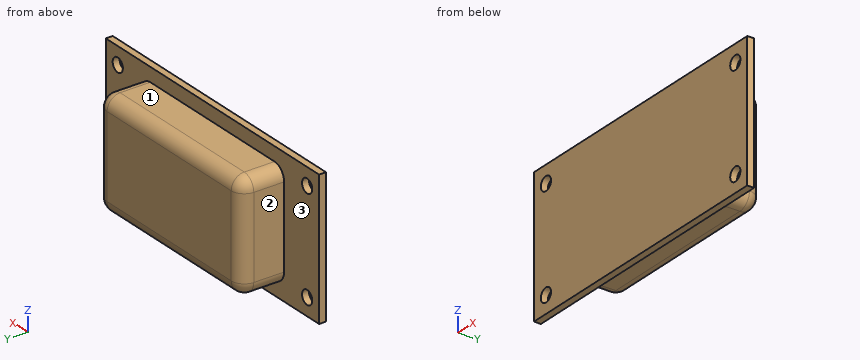
```python
from build123d import *

# Parameters (mm, degrees)
SKETCH_1_W      = 67
SKETCH_1_H      = 31.5
SKETCH_1_R      = 1.6
EXTRUDE_1_DEPTH = 1.6
SKETCH_2_W      = 45
SKETCH_2_H      = 25
EXTRUDE_2_DEPTH = 10
FILLET_1_R      = 3


with BuildPart() as part:
    # 草圖1 → 填料-伸長1 (new body)
    with BuildSketch(Plane(origin=(0, 0, 0), x_dir=(1, 0, 0), z_dir=(0, 1, 0))):
        Rectangle(SKETCH_1_W, SKETCH_1_H)
        with Locations(Location((-29.75, 11.75, 0), (0, 0, 270))):
            Circle(SKETCH_1_R, mode=Mode.SUBTRACT)
        with Locations(Location((-29.75, -11.75, 0), (0, 0, 270))):
            Circle(SKETCH_1_R, mode=Mode.SUBTRACT)
        with Locations(Location((29.75, -11.75, 0), (0, 0, 270))):
            Circle(SKETCH_1_R, mode=Mode.SUBTRACT)
        with Locations(Location((29.75, 11.75, 0), (0, 0, 270))):
            Circle(SKETCH_1_R, mode=Mode.SUBTRACT)
    extrude(amount=EXTRUDE_1_DEPTH)

    # 草圖2 → 填料-伸長2 (add)
    with BuildSketch(Plane(origin=(0, 1.6, 0), x_dir=(1, 0, 0), z_dir=(0, 1, 0))):
        Rectangle(SKETCH_2_W, SKETCH_2_H)
    extrude(amount=EXTRUDE_2_DEPTH)

    # 圓角1
    fillet_1_edges = [part.edges().sort_by_distance(p)[0] for p in [
        (22.5, 6.6, 12.5),
        (22.5, 6.6, -12.5),
        (-22.5, 6.6, -12.5),
        (-22.5, 6.6, 12.5),
        (22.5, 11.6, 0),
        (0, 11.6, -12.5),
        (-22.5, 11.6, 0),
        (0, 11.6, 12.5),
    ]]
    fillet(fillet_1_edges, radius=FILLET_1_R)


solid = part.part
```
Model file for the job. Use its own axes, mm. Face numbers are marked on the shaded views. A direction names the side the tool comes from. Coordinates: 2 decimals unless noted, no trailing zeros. Write each loop counter-clockwise with the first axis right and the second up, starting at its lowest first coordinate (ties: lowest second). Pieces come first, ordered by that corner, then holes. Notation, with made-up numbers: (2.5, -2) - (15.5, -2) arc R23 cw to (15.5, 11) - close; hole circle Ø9 at (-26.5, 16). An arc over 180 degrees is marked (long way). One line per item, written item: value. Start each with the question number.
1. Flat gauge pins, fed straight in: pin 1 (1 mm diameter, centred on y = 5, z = 4, fed in from +X); pin 2 (6 mm diameter, centred on x = 7.5, y = 7, fed in from -Z); pin 3 (5.5 mm diameter, centred on y = 5.5, z = -0.5, fed in from -X). Where does each tip first touch, or does it go through?
2. Slice it at A-A (x = 29.75). Write the cut outline in (y, z), plus the area to 3 significant figures.
3. Slice it at C-C (z = 11.75). Write the cut outline in (x, y), plus the area to 3 significant figures.
4. Probe line 1 (X direction, y = 1, z = 11.75); line 2 (Z direction, x = -29.5, y = 1.25); line 3 (Z direction, x = 13, y = 7.5). List the from-to ranges inside material, lowest first. Write a range as from..to.
5. Slice it at B-B (y = 1). Write the cut outline in (x, z), plus the area to 3 significant figures.
6. Tool access for the marked faces 1, 2 and 3: list every direction of +Z, -Z, +X, -X, +Y, -Y with a clear straight run to the whole face (end or side of a thin tool).
7. Slice it at D-D (y = 4.5). Write the cut outline in (x, z), plus the area to 3 significant figures.
Answers below:
1. pin 1: stops at x = 22.5
1. pin 2: stops at z = -12.5
1. pin 3: stops at x = -22.5
2. outline: (0, -15.75) - (1.6, -15.75) - (1.6, -13.35) - (0, -13.35) - close; (0, -10.15) - (1.6, -10.15) - (1.6, 10.15) - (0, 10.15) - close; (0, 13.35) - (1.6, 13.35) - (1.6, 15.75) - (0, 15.75) - close
2. area: 40.2 mm^2
3. outline: (-33.5, 0) - (-31.35, 0) - (-31.35, 1.6) - (-33.5, 1.6) - close; (-28.15, 0) - (28.15, 0) - (28.15, 1.6) - (21.48, 1.6) - (21.48, 8.6) arc R1.98 ccw to (19.5, 10.58) - (-19.5, 10.58) arc R1.98 ccw to (-21.48, 8.6) - (-21.48, 1.6) - (-28.15, 1.6) - close; (31.35, 0) - (33.5, 0) - (33.5, 1.6) - (31.35, 1.6) - close
3. area: 481 mm^2
4. line 1: x = -33.5..-31.35, -28.15..28.15, 31.35..33.5
4. line 2: z = -15.75..-13.33, -10.17..10.17, 13.33..15.75
4. line 3: z = -12.5..12.5
5. outline: (-33.5, -15.75) - (33.5, -15.75) - (33.5, 15.75) - (-33.5, 15.75) - close; hole circle Ø3.2 at (-29.75, -11.75); hole circle Ø3.2 at (-29.75, 11.75); hole circle Ø3.2 at (29.75, -11.75); hole circle Ø3.2 at (29.75, 11.75)
5. area: 2,080 mm^2
6. face 1: +Z, +X, -X, +Y
6. face 2: +Z, -Z, -X, +Y
6. face 3: +Y
7. outline: (-22.5, -9.5) arc R3 ccw to (-19.5, -12.5) - (19.5, -12.5) arc R3 ccw to (22.5, -9.5) - (22.5, 9.5) arc R3 ccw to (19.5, 12.5) - (-19.5, 12.5) arc R3 ccw to (-22.5, 9.5) - close
7. area: 1,120 mm^2
